from build123d import *

# Parameters (mm, degrees)
SKETCH1_R           = 1.905
BOSS_EXTRUDE1_DEPTH = 2.413
SKETCH3_W           = 34
SKETCH3_H           = 30
SKETCH3_R           = 1.905
BOSS_EXTRUDE2_DEPTH = 4.064
FILLET1_R           = 5
SKETCH5_W           = 13.68
SKETCH5_H           = 4.826
SKETCH5_H_2         = 1.087
BOSS_EXTRUDE4_DEPTH = 5
SKETCH5_3_W         = 13.68
SKETCH5_3_H         = 4
BOSS_EXTRUDE5_DEPTH = 20
CUT_EXTRUDE1_REACH  = 69.799
SKETCH6_R           = 1.5
FILLET2_R           = 3


with BuildPart() as part:
    # Sketch1 → Boss-Extrude1 (new, symmetric)
    # profile 1 of 2: a face of its own
    with BuildSketch(Plane.XY):
        Polygon((-17, 31.496), (-17, 0), (17, 0), (17, 31.496), (6.84, 31.496), (6.84, 41.656), (-6.84, 41.656), (-6.84, 31.496), align=None)
        with Locations((0, 5.207)):
            Circle(SKETCH1_R, mode=Mode.SUBTRACT)
        with Locations((0, 36.449)):
            Circle(SKETCH1_R, mode=Mode.SUBTRACT)
    # profile 2 of 2: a face of its own
    with BuildSketch(Plane.XY):
        Polygon((-17, 31.496), (-17, 0), (17, 0), (17, 31.496), (6.84, 31.496), (6.84, 41.656), (-6.84, 41.656), (-6.84, 31.496), align=None)
        with Locations((0, 5.207)):
            Circle(SKETCH1_R, mode=Mode.SUBTRACT)
        with Locations((0, 36.449)):
            Circle(SKETCH1_R, mode=Mode.SUBTRACT)
    extrude(amount=BOSS_EXTRUDE1_DEPTH, both=True)

    # Sketch3 → Boss-Extrude2 (add)
    with BuildSketch(Plane(origin=(0, 0, 0), x_dir=(1, 0, 0), z_dir=(0, 1, 0))):
        Rectangle(SKETCH3_W, SKETCH3_H)
        with Locations(Location((-11.935, -9.11, 0), (0, 0, 270))):
            Circle(SKETCH3_R, mode=Mode.SUBTRACT)
        with Locations(Location((11.935, -9.11, 0), (0, 0, 270))):
            Circle(SKETCH3_R, mode=Mode.SUBTRACT)
        with Locations(Location((11.935, 9.11, 0), (0, 0, 270))):
            Circle(SKETCH3_R, mode=Mode.SUBTRACT)
        with Locations(Location((-11.935, 9.11, 0), (0, 0, 270))):
            Circle(SKETCH3_R, mode=Mode.SUBTRACT)
    extrude(amount=-BOSS_EXTRUDE2_DEPTH)

    # Fillet1
    fillet1_edges = [part.edges().sort_by_distance(p)[0] for p in [
        (6.84, 31.496, 0),
        (17, 31.496, 0),
        (-17, 31.496, 0),
        (-6.84, 31.496, 0),
    ]]
    fillet(fillet1_edges, radius=FILLET1_R)

    # Sketch5 → Boss-Extrude4 (add)
    with BuildSketch(Plane(origin=(0, 41.656, 0), x_dir=(1, 0, 0), z_dir=(0, 1, 0))):
        Rectangle(SKETCH5_W, SKETCH5_H)
        with Locations((0, -2.9565)):
            Rectangle(SKETCH5_W, SKETCH5_H_2)
        with Locations((0, 2.9565)):
            Rectangle(SKETCH5_W, SKETCH5_H_2)
    extrude(amount=BOSS_EXTRUDE4_DEPTH)

    # Sketch5<3> → Boss-Extrude5 (add)
    with BuildSketch(Plane(origin=(0, 41.656, 0), x_dir=(1, 0, 0), z_dir=(0, 1, 0))):
        with Locations((0, -5.5)):
            Rectangle(SKETCH5_3_W, SKETCH5_3_H)
        with Locations((0, 5.5)):
            Rectangle(SKETCH5_3_W, SKETCH5_3_H)
    extrude(amount=BOSS_EXTRUDE5_DEPTH)

    # Cut-Extrude1: up to this face of the body (flat: up to its plane)
    cut_extrude1_end = Plane(part.part.faces().sort_by_distance((0, 51.656, 7.5))[0])
    # Sketch6 → Cut-Extrude1 (cut, up to the picked face)
    with BuildSketch(Plane(origin=(0, 0, -7.5), x_dir=(-1, 0, 0), z_dir=(0, 0, -1)), mode=Mode.PRIVATE) as cut_extrude1_sk1:
        with Locations((0, 55.656)):
            Circle(SKETCH6_R)
    cut_extrude1_tool1 = split(extrude(cut_extrude1_sk1.sketch, amount=-CUT_EXTRUDE1_REACH, mode=Mode.PRIVATE), bisect_by=cut_extrude1_end, keep=Keep.BOTH, mode=Mode.PRIVATE)
    add(cut_extrude1_tool1.solids().sort_by(Axis((0, 55.656, -7.5), (0, 0, 1)))[0], mode=Mode.SUBTRACT)

    # Fillet2
    fillet2_edges = [part.edges().sort_by_distance(p)[0] for p in [
        (0, 41.656, -7.5),
        (0, 46.656, -3.5),
        (0, 46.656, 3.5),
        (0, 41.656, 7.5),
    ]]
    fillet(fillet2_edges, radius=FILLET2_R)


solid = part.part
The model under review builds one solid part; all positions refer to its coordinate system, in mm. A direction names the side the tool comes from. Round coordinates to 2 decimals unless told otherwise and drop trailing zeros. Write each loop counter-clockwise with the first axis right and the second up, starting at its lowest first coordinate (ties: lowest second). Pieces come first, ordered by that corner, then holes. Notation, with made-up numbers: M -12.75,73 L 35.25,73 A26 cw 35.25,92 Z; hole C -34,-30 d1. An arc over 180 degrees is marked long. Answer as CSV lines item,"result". Start each with the question number.
Q1. Consider section B-B, the plane z = 9.11. Give the boundary of the cut face in (x, y), then the cut area to 3 significant figures.
Q2. Consider section C-C, the plane x = -4.5. Give the boundary of the cut face in (y, z), then the cut area to 3 significant figures.
Q3. The part is to be moulded in two halves that separate along Y. For faces 5 (the face through (0.195, 57.143, -5.528)), 6 (the face through (-6.84, 46, 0)), 7 (the face through (0, 41.656, -3)), 8 (the face through (0, 61.656, -6)), say which applies: +Y half, -Y half, draft (parallel to the pull), parting line (faces both ways), or undercut.
Q4. Tool access review of faces 1 (the face through (0, 48, -3)), 2 (the face through (-12.66, -2, 10.87)), 3 (the face through (0, 16, 2.413)), 4 (the face through (0, 0, -9)): name each direction out of +Z, -Z, +X, -X, +Y, -Y from which nothing blocks a thin tool from reaching the whole face with its end or side.
Q5. Wall thickness on line 1 along Y through (x, z) = (0, -0.5); line 2 along Y through (x, z) = (0, -6.25); line 3 along X through (y, z) = (-2.7, 9.11): over which ranges is each line inside the solid? List them lowest first.
Q6. Consider section A-A, the plane y = 52. Give the boundary of the cut face in (x, z).
Q7. Consider section D-D, the plane z = 5.75. Give the boundary of the cut face in (x, y), then the cut area to 3 significant figures.
Q8. Clearance check with flat-ended pins moving along their axes: P1, Ø17, axis at x = 1, y = 28.5, coming from the +Z side; P2, Ø16.5, axis at y = 43.5, z = 2, coming from the -X side; P3, Ø8, axis at x = 3, y = 50, coming from the +Z side; P4, Ø12, axis at x = -3.5, z = 11.5, coming from the +Y side. State where each tip first meets the part, or that it passes through.
Result set:
1,outline,"M -17,-4.06 L -13.84,-4.06 L -13.84,0 L -17,0 Z; M -10.03,-4.06 L 10.03,-4.06 L 10.03,0 L -10.03,0 Z; M 13.84,-4.06 L 17,-4.06 L 17,0 L 13.84,0 Z"
1,area,"107 mm²"
2,outline,"M -4.06,-15 L 0,-15 L 0,-2.41 L 41.66,-2.41 L 41.66,-4.5 A3 ccw 44.66,-7.5 L 61.66,-7.5 L 61.66,-3.5 L 49.66,-3.5 A3 cw 46.66,-0.5 L 46.66,0.5 A3 cw 49.66,3.5 L 61.66,3.5 L 61.66,7.5 L 44.66,7.5 A3 ccw 41.66,4.5 L 41.66,2.41 L 0,2.41 L 0,15 L -4.06,15 Z"
2,area,"518 mm²"
3,face 5,"undercut"
3,face 6,"draft"
3,face 7,"undercut"
3,face 8,"+Y half"
4,face 1,"+X, -X, +Y"
4,face 2,"+Y, -Y"
4,face 3,"+Z, +X, -X"
4,face 4,"-Z, +X, -X"
5,line 1,"y = -4.06 to 3.3, 7.11 to 34.54, 38.35 to 46.66"
5,line 2,"y = -4.06 to 0, 42.22 to 54.16, 57.16 to 61.66"
5,line 3,"x = -17 to -13.84, -10.03 to 10.03, 13.84 to 17"
6,outline,"M -6.84,-7.5 L 6.84,-7.5 L 6.84,-3.5 L -6.84,-3.5 Z; M -6.84,3.5 L 6.84,3.5 L 6.84,7.5 L -6.84,7.5 Z"
7,outline,"M -17,-4.06 L 17,-4.06 L 17,0 L -17,0 Z; M -6.84,41.93 L 6.84,41.93 L 6.84,61.66 L -6.84,61.66 Z; hole C 0,55.66 d3"
7,area,"401 mm²"
8,P1,"stops at z = 2.41"
8,P2,"stops at x = -7"
8,P3,"stops at z = 7.5"
8,P4,"stops at y = 61.66"
